Could you check a few things on this model? Use its own coordinates, in mm. Round coordinates to 2 decimals unless told otherwise and drop trailing zeros. Write each loop counter-clockwise with the first axis right and the second up, starting at its lowest first coordinate (ties: lowest second). Pieces come first, ordered by that corner, then holes. Notation, with made-up numbers: M 81,-39.5 L 117,-39.5 A18 cw 117,-8.5 Z; hole C 24.25,-27.75 d10. An arc over 180 degrees is marked long. One line per item, written item: value. Start each with the question number.
(1) I want a section at A-A on z = 2.5. Please give me the cut outline in (x, y), and give its area (3 significant figures).
(2) I want a section at B-B on x = 18. Please give me the cut outline in (y, z), and give its area (3 significant figures).
(3) I'm going to push flat-ended pins straight in: pin 1 Ø0.7 at (y, z) = (0.5, 3.5) entering from -X; pin 2 Ø1.5 at (x, z) = (12.5, 1.5) entering from -Y. Where does each tip first touch, or does it pass through?
(4) If I drill on L1, parallel to Z at x = 17, y = 0.1; L2, parallel to X at y = 0.55, z = 4.75, over which ranges is the centre line in solid material (lowest first)?
```python
from build123d import *
from OCP.BRepFilletAPI import BRepFilletAPI_MakeFillet

# Parameters (mm, degrees)
BOSS_EXTRUDE1_DEPTH = 1.32
FILLET1_R           = 3
FILLET2_R           = 2.6
FILLET3_R1          = 1.2
FILLET3_R2          = 1
FILLET4_R           = 0.4
FILLET5_R           = 1.8
FILLET6_R           = 1.6


with BuildPart() as part:
    # Sketch1 → Boss-Extrude1 (new body)
    with BuildSketch(Plane(origin=(0, 0, 0), x_dir=(1, 0, 0), z_dir=(0, 1, 0))):
        Polygon((0, 0), (2.92, 0), (2.92, -7.77), (9.82, -7.77), (9.82, -5.85), (19.92, -5.85), (19.92, -7.77), (26.82, -7.77), (26.82, 5.05), (0, 5.05), align=None)
    extrude(amount=BOSS_EXTRUDE1_DEPTH)

    # Fillet1
    fillet1_edges = [part.edges().sort_by_distance(p)[0] for p in [
        (26.82, 0.66, -5.05),
        (2.92, 0.66, 7.77),
    ]]
    fillet(fillet1_edges, radius=FILLET1_R)

    # Fillet2
    fillet2_edges = [part.edges().sort_by_distance(p)[0] for p in [
        (26.82, 0.66, 7.77),
    ]]
    fillet(fillet2_edges, radius=FILLET2_R)

    # Fillet3: one fillet with a radius per group of edges: ONE call of the kernel's fillet builder (fillet() takes one radius for all edges)
    fillet3_edges_1 = [part.edges().sort_by_distance(p)[0] for p in [
        (19.92, 0.66, 7.77),
    ]]
    fillet3_edges_2 = [part.edges().sort_by_distance(p)[0] for p in [
        (9.82, 0.66, 7.77),
    ]]
    fillet3 = BRepFilletAPI_MakeFillet(part.part.solid().wrapped)
    for e in fillet3_edges_1:
        fillet3.Add(FILLET3_R1, e.wrapped)
    for e in fillet3_edges_2:
        fillet3.Add(FILLET3_R2, e.wrapped)
    add(Compound.cast(fillet3.Shape()), mode=Mode.REPLACE)

    # Fillet4
    fillet4_edges = [part.edges().sort_by_distance(p)[0] for p in [
        (19.92, 0.66, 5.85),
        (9.82, 0.66, 5.85),
    ]]
    fillet(fillet4_edges, radius=FILLET4_R)

    # Fillet5
    fillet5_edges = [part.edges().sort_by_distance(p)[0] for p in [
        (0, 0.66, -5.05),
        (0, 0.66, 0),
    ]]
    fillet(fillet5_edges, radius=FILLET5_R)

    # Fillet6
    fillet6_edges = [part.edges().sort_by_distance(p)[0] for p in [
        (2.92, 0.66, 0),
    ]]
    fillet(fillet6_edges, radius=FILLET6_R)


solid = part.part
```
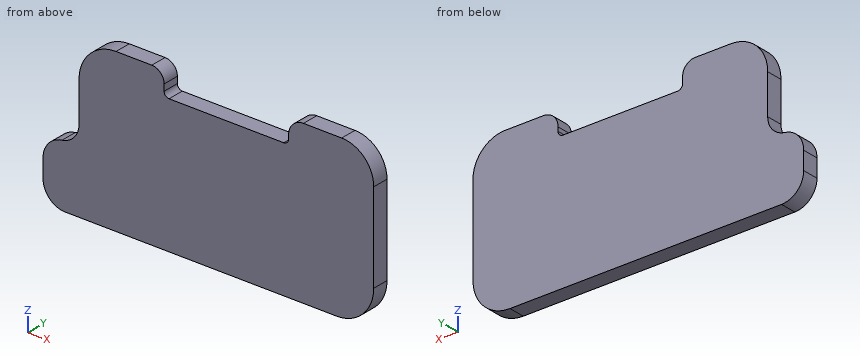
Found:
1. outline: M 2.92,0 L 26.82,0 L 26.82,1.32 L 2.92,1.32 Z
1. area: 31.5 mm²
2. outline: M 0,-5.05 L 1.32,-5.05 L 1.32,5.85 L 0,5.85 Z
2. area: 14.4 mm²
3. pin 1: stops at x = 2.92
3. pin 2: stops at y = 0
4. L1: z = -5.05 to 5.85
4. L2: x = 2.92 to 26.82
